Input: dimensioned drawing with shaded views. Units: mm. Origin: part minimum x, y, z. Round coordinates to 2 decimals unless told otherwise and drop trailing zeros. Write each loop counter-clockwise with the first axis right and the second up, starting at its lowest first coordinate (ties: lowest second). Pieces come first, ordered by that corner, then holes. Notation, with made-up numbers: (14, 18.5) -> (37, 18.5) arc R17 cw to (37, 50.5) -> close; hole circle Ø6 at (52, 17). An arc over 180 degrees is marked (long way). Use one line per item in the form item = value. Start each with the question number.
1. Line query: L1, parallel to X at y = 153, z = 2.75 (1 decimal); L2, parallel to Y at x = 5, z = 5.75. Output: solid intervals per line, ascending.
2. Cut plane B-B, the plane y = 207. Return the cut outline in (x, z) (1 decimal).
3. Pin query (flat end, axial travel): pin 1 Ø1.5 at (y, z) = (68.5, 8.5) entering from +X (1 decimal); pin 2 Ø1.5 at (y, z) = (48.5, 3) entering from -X (1 decimal); pin 3 Ø5 at (x, z) = (41.5, 4) entering from -Y; pin 4 Ø8 at (x, y) = (26.5, 90) entering from -Z. Return the tip coordinate at first contact, or that it passes through.
4. Cut plane C-C, the plane x = 42. Return the cut outline in (y, z).
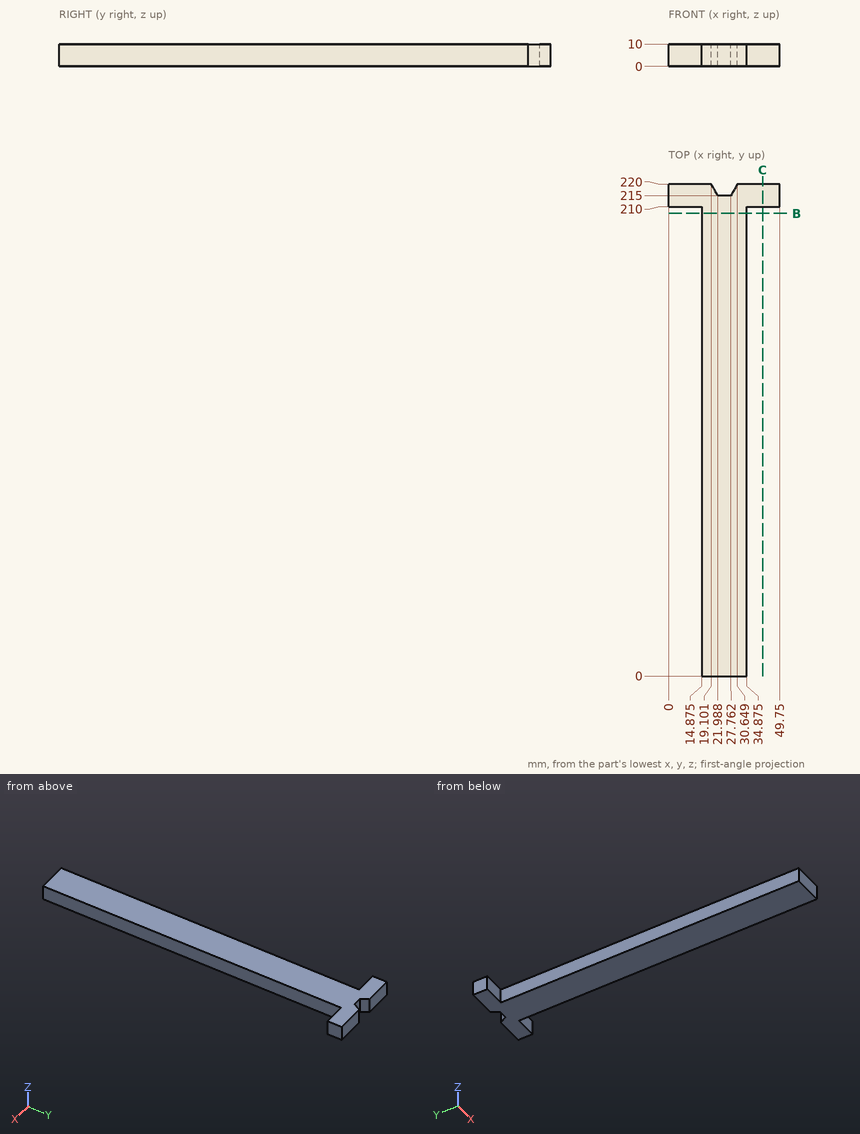
Outcome:
q1.L1 = 14.9 to 34.9
q1.L2 = 210 to 220
q2.outline = (14.9, 0) -> (34.9, 0) -> (34.9, 10) -> (14.9, 10) -> close
q3.pin_1 = 34.9
q3.pin_2 = 14.9
q3.pin_3 = 210
q3.pin_4 = 0
q4.outline = (210, 0) -> (220, 0) -> (220, 10) -> (210, 10) -> close
